Build history of the part. All positions in model axes, mm. Face numbers are marked on the shaded views. A direction names the side the tool comes from. Round coordinates to 2 decimals unless told otherwise and drop trailing zeros. Write each loop counter-clockwise with the first axis right and the second up, starting at its lowest first coordinate (ties: lowest second). Pieces come first, ordered by that corner, then holes. Notation, with made-up numbers: (33, 73.25) - (46, 73.25) arc R27 cw to (46, 108.25) - close; hole circle Ø1 at (82.25, -5). An arc over 180 degrees is marked (long way). Answer as a JSON object with one key per item and string values. Group by question number.
Item 1: Two-plate mould, pull along X, no slides. Class the marked faces 1, 2 and 3: +X half, -X half, draft (parallel to the pull), parting line (faces both ways), or undercut.
Item 2: Which spindle directions (+Z, -Z, +X, -X, +Y, -Y) get a long thin tool onto all of the face, cutting with end or side? Do the marked faces 4, 5, 6 and 7. Say none if no direction does.
Item 3: Slice it at C-C, the plane y = -14.5. List the corners of the cut face in (x, z), then the cut area to 3 significant figures.
Item 4: Slice it at D-D, the plane y = -25. List the corners of the cut face in (x, z).
Item 5: Slice it at A-A, the plane z = 0. List the corners of the cut face in (x, y).
Item 6: Probe line 1 (X direction, y = 3.65, z = -15.5); line 2 (X direction, y = -12, z = 2.5); line 3 (X direction, y = -7.75, z = 64). List the from-to ranges inside material, lowest first. Write a range as from..to.
Item 7: Flat gauge pins, fed straight in: pin 1 (12 mm diameter, centred on y = -13, z = 18, fed in from +X); pin 2 (10 mm diameter, centred on x = 24, y = -4.5, fed in from +Z); pin 3 (16.5 mm diameter, centred on x = 10, y = -10, fed in from -Z); pin 4 (4 mm diameter, centred on x = -15.5, z = 15.5, fed in from +Y). Where does each tip first touch, or does it go through?
Item 8: Slice it at B-B, the plane x = 40. List the corners of the cut face in (y, z).
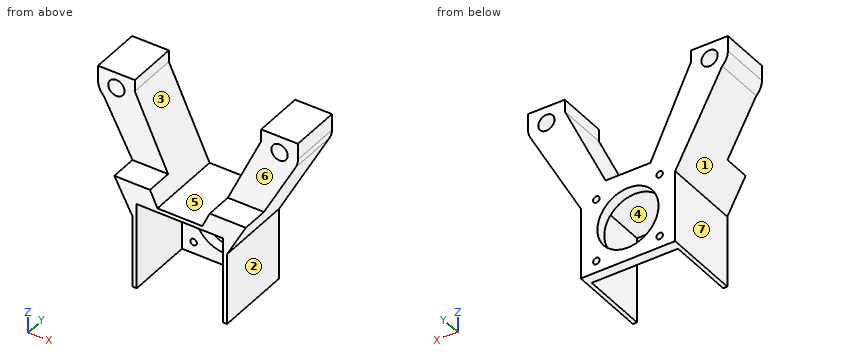
from build123d import *

# Parameters (mm, degrees)
SKETCH_6_W          = 42.3
SKETCH_6_H          = 42.3
SKETCH_6_R          = 1.6
SKETCH_6_R_2        = 15
EXTRUDE_1_DEPTH     = 5
SKETCH_7_R          = 4
EXTRUDE_5_DEPTH     = 38
EXTRUDE_START       = 38
SKETCH_7_7_R        = 4
EXTRUDE_7_DEPTH     = 38
SKETCH_7_8_R        = 4
EXTRUDE_8_DEPTH     = 38
SKETCH_12_W         = 2
SKETCH_12_H         = 44.3
EXTRUDE_11_DEPTH    = 38
SKETCH_14_W         = 44.3
SKETCH_14_H         = 2
EXTRUDE_12_DEPTH    = 38
SKETCH_15_W         = 2
SKETCH_15_H         = 42.3
EXTRUDE_13_DEPTH    = 38
CUT_EXTRUDE_1_DEPTH = 13.2


with BuildPart() as part:
    # 草图6 → 凸台-拉伸1 (new body)
    with BuildSketch(Plane(origin=(0, 0, 0), x_dir=(1, 0, 0), z_dir=(0, 1, 0))):
        Rectangle(SKETCH_6_W, SKETCH_6_H)
        with Locations(Location((15.5, 15.5, 0), (0, 0, 270))):
            Circle(SKETCH_6_R, mode=Mode.SUBTRACT)
        with Locations(Location((-15.5, 15.5, 0), (0, 0, 270))):
            Circle(SKETCH_6_R, mode=Mode.SUBTRACT)
        with Locations(Location((-15.5, -15.5, 0), (0, 0, 270))):
            Circle(SKETCH_6_R, mode=Mode.SUBTRACT)
        with Locations(Location((15.5, -15.5, 0), (0, 0, 270))):
            Circle(SKETCH_6_R, mode=Mode.SUBTRACT)
        with Locations(Location((0, 0, 0), (0, 0, 270))):
            Circle(SKETCH_6_R_2, mode=Mode.SUBTRACT)
    extrude(amount=EXTRUDE_1_DEPTH)

    # 草图7 → 凸台-拉伸5 (add)
    # profile 1 of 2: a face of its own
    with BuildSketch(Plane(origin=(0, 5, 0), x_dir=(1, 0, 0), z_dir=(0, 1, 0))):
        with BuildLine():
            Line((49, -72), (49, -64))
            ThreePointArc((49, -64), (48.724429591, -61.789948347), (47.914593709, -59.715235547))
            Line((47.914593709, -59.715235547), (21.15, -10.277072187))
            Line((21.15, -10.277072187), (21.15, -21.15))
            Line((21.15, -21.15), (10.070005019, -21.15))
            Line((10.070005019, -21.15), (30.963898233, -65.919418373))
            Line((30.963898233, -65.919418373), (30.963898233, -71.907979073))
            Line((30.963898233, -71.907979073), (49, -72))
        make_face()
        with Locations(Location((40, -64, 0), (0, 0, 270))):
            Circle(SKETCH_7_R, mode=Mode.SUBTRACT)
    # profile 2 of 2: a face of its own
    with BuildSketch(Plane(origin=(0, 5, 0), x_dir=(1, 0, 0), z_dir=(0, 1, 0))):
        with BuildLine():
            Line((-30.963898233, -65.919418373), (-10.070005019, -21.15))
            Line((-10.070005019, -21.15), (-21.15, -21.15))
            Line((-21.15, -21.15), (-21.15, -10.282583808))
            Line((-21.15, -10.282583808), (-46.202269248, -57.478354795))
            ThreePointArc((-46.202269248, -57.478354795), (-48.271046585, -60.45179082), (-49, -64))
            Line((-49, -64), (-49, -71.5))
            Line((-49, -71.5), (-30.963898233, -71.592020927))
            Line((-30.963898233, -71.592020927), (-30.963898233, -65.919418373))
        make_face()
        with Locations(Location((-40, -64, 0), (0, 0, 270))):
            Circle(SKETCH_7_R, mode=Mode.SUBTRACT)
    extrude(amount=-EXTRUDE_5_DEPTH)

    # 草图7<7> → 凸台-拉伸7 (add)
    with BuildSketch(Plane(origin=(0, 5, 0), x_dir=(1, 0, 0), z_dir=(0, 1, 0)).offset(EXTRUDE_START)):
        with Locations(Location((-40, -64, 0), (0, 0, 270))):
            Circle(SKETCH_7_7_R)
        with Locations(Location((40, -64, 0), (0, 0, 270))):
            Circle(SKETCH_7_7_R)
    extrude(amount=-EXTRUDE_7_DEPTH)


with BuildPart() as extrude_7_kept_piece:
    # of the separate pieces the step leaves, the one the design keeps (extrude_7_pieces_kept)
    add(part.part.solids().sort_by_distance((-10.070005019, 0, 21.15))[0])

    # 草图7<8> → 凸台-拉伸8 (add)
    with BuildSketch(Plane(origin=(0, 5, 0), x_dir=(1, 0, 0), z_dir=(0, 1, 0))):
        with Locations(Location((-40, -64, 0), (0, 0, 270))):
            Circle(SKETCH_7_8_R)
        with Locations(Location((40, -64, 0), (0, 0, 270))):
            Circle(SKETCH_7_8_R)
    extrude(amount=EXTRUDE_8_DEPTH)


with BuildPart() as extrude_8_kept_piece:
    # of the separate pieces the step leaves, the one the design keeps (extrude_8_pieces_kept)
    add(extrude_7_kept_piece.part.solids().sort_by_distance((-10.070005019, 0, 21.15))[0])

    # 草图12 → 凸台-拉伸11 (add)
    with BuildSketch(Plane(origin=(0, 5, 0), x_dir=(1, 0, 0), z_dir=(0, 1, 0))):
        with Locations((22.15, -1)):
            Rectangle(SKETCH_12_W, SKETCH_12_H)
    extrude(amount=-EXTRUDE_11_DEPTH)

    # 草图14 → 凸台-拉伸12 (add)
    with BuildSketch(Plane(origin=(0, 5, 0), x_dir=(1, 0, 0), z_dir=(0, 1, 0))):
        with Locations((-1, -22.15)):
            Rectangle(SKETCH_14_W, SKETCH_14_H)
    extrude(amount=-EXTRUDE_12_DEPTH)

    # 草图15 → 凸台-拉伸13 (add)
    with BuildSketch(Plane(origin=(0, 5, 0), x_dir=(1, 0, 0), z_dir=(0, 1, 0))):
        with Locations((-22.15, 0)):
            Rectangle(SKETCH_15_W, SKETCH_15_H)
    extrude(amount=-EXTRUDE_13_DEPTH)

    # 草图17 → 切除-拉伸1 (cut)
    with BuildSketch(Plane.XZ.offset(33)):
        Polygon((62.040525686, 30.953335803), (-8.604799232, 30.953335803), (-61.83718559, 30.953335803), (-61.83718559, 85.06296978), (-8.604799232, 85.06296978), (62.040525686, 85.06296978), align=None)
    extrude(amount=-CUT_EXTRUDE_1_DEPTH, mode=Mode.SUBTRACT)


solid = extrude_8_kept_piece.part
Geometry says:
{
 "1": {"face 1": "-X half", "face 2": "+X half", "face 3": "undercut"},
 "2": {"face 4": "-Z, -Y", "face 5": "+Z, +Y, -Y", "face 6": "+Z, +X, -X, -Y", "face 7": "-Z, -X, +Y, -Y"},
 "3": {"outline": "(-49, 64) arc R9 ccw to (-46.2, 57.48) - (-23.15, 14.05) - (-23.15, -21.15) - (-21.15, -21.15) - (-21.15, 21.15) - (21.15, 21.15) - (21.15, -21.15) - (23.15, -21.15) - (23.15, 13.97) - (47.91, 59.72) arc R9 ccw to (49, 64) - (49, 72) - (30.96, 71.91) - (30.96, 65.92) - (11, 23.15) - (-11, 23.15) - (-30.96, 65.92) - (-30.96, 71.59) - (-49, 71.5) - close; hole circle Ø8 at (-40, 64); hole circle Ø8 at (40, 64)", "area": "2,000 mm^2"},
 "4": {"outline": "(-32.12, 30.95) - (-23.15, 14.05) - (-23.15, -21.15) - (-21.15, -21.15) - (-21.15, 21.15) - (21.15, 21.15) - (21.15, -21.15) - (23.15, -21.15) - (23.15, 13.97) - (32.34, 30.95) - (14.65, 30.95) - (11, 23.15) - (-11, 23.15) - (-14.65, 30.95) - close"},
 "5": {"outline": "(-23.15, -33) - (-21.15, -33) - (-21.15, 0) - (-15, 0) - (-15, 5) - (-23.15, 5) - close; (15, 0) - (21.15, 0) - (21.15, -33) - (23.15, -33) - (23.15, 5) - (15, 5) - close"},
 "6": {"line 1": "x = -23.15..-17.1, -13.9..13.9, 17.1..23.15", "line 2": "x = -23.15..-21.15, 21.15..23.15", "line 3": "x = -49..-44, -36..-30.07, 30.07..36, 44..49"},
 "7": {"pin 1": "stops at x = 28.58", "pin 2": "stops at z = 61.71", "pin 3": "stops at z = 21.15", "pin 4": "stops at y = 5"},
 "8": {"outline": "(-19.8, 45.1) - (5, 45.1) - (5, 60) - (-19.8, 60) - close; (-19.8, 68) - (5, 68) - (5, 71.95) - (-19.8, 71.95) - close"}
}
